Geometry: final body of the model. Coordinates: model frame, mm. A direction names the side the tool comes from. Round coordinates to 2 decimals unless told otherwise and drop trailing zeros. Order: outer loops, then holes, each group sorted by start corner. A loop starts at its lowest first (then second) coordinate and runs counter-clockwise, first axis right, second up. Notation, with made-up numbers: (-27, 54.25) - (22, 54.25) arc R7 cw to (22, 67.25) - close; hole circle Ø10 at (-12, -36). An arc over 180 degrees is marked (long way). Put each result on its own line as item: value. Start each with the question number.
(1) Access query for faces 4 (the face through (208, 44, 6)), 5 (the face through (411.7, 106.6, 3)). Directions: +Z, -Z, +X, -X, +Y, -Y. A direction counts if a zero-diameter tool reaches every point of the face in a straight line with its end or side. Return the directions, or none.
(2) Pull-direction query (X, two-part tool) for faces 1 (the face through (334.87, 80.88, 2.96)), 2 (the face through (443.46, 91.16, 2.96)), 3 (the face through (-72.19, 134.884, 2.958)); classes: released by +X, released by -X, zero draft, split by the parting line, or undercut.
(3) Pin query (flat end, axial travel): P1, Ø1, axis at x = 92, z = 3, coming from the -Y side; P2, Ø2, axis at y = 35, z = 4, coming from the -X side; P3, Ø1.5, axis at x = 399.5, z = 2, coming from the -Y side. Return the tip coordinate at first contact, or that it passes through.
(4) Material intervals for L1, parallel to Y at x = 436.5, z = 2.75; L2, parallel to X at y = 141, z = 2; L3, parallel to X at y = 142, z = 4, sorted ascending. Write a range as [from, to].
(5) Section A-A (x = 363). Output: boundary loops of the cut face in (y, z), and give its area (3 significant figures).
(6) Section B-B (y = 143.5). Output: boundary loops of the cut face in (x, z).
from build123d import *

# Parameters (mm, degrees)
BOSS_EXTRU_3_DEPTH = 6
CONG_1_R           = 60


with BuildPart() as part:
    # Esquisse3 → Boss.-Extru.3 (new body)
    with BuildSketch(Plane(origin=(-3.638307048, 7.762911288, 0), x_dir=(0.984807753012208, -0.1736481776669307, 0), z_dir=(0, 0, 1))):
        with BuildLine():
            Line((-71.559692406, 137.419515489), (-65.127612513, 98.953577983))
            Line((-65.127612513, 98.953577983), (-46.578471081, 103.06810738))
            Line((-46.578471081, 103.06810738), (-41.164616612, 78.661342338))
            Line((-41.164616612, 78.661342338), (-38.235804807, 79.311004874))
            Line((-38.235804807, 79.311004874), (-40.632352311, 90.115131983))
            Line((-40.632352311, 90.115131983), (-35.750999303, 91.197902877))
            Line((-35.750999303, 91.197902877), (-20.829774243, 61.686423244))
            add(Edge.make_bspline(
                [(38.37456384, 38.513359507), (16.587805448, 35.939302498), (-7.762740615, 43.297007319), (-20.829774243, 61.686423244)],
                knots=[0, 0, 0, 0, 1, 1, 1, 1], degree=3))
            Line((38.37456384, 38.513359507), (40.525402219, 28.816939468))
            Line((40.525402219, 28.816939468), (43.463887608, 29.421342988))
            Line((43.463887608, 29.421342988), (41.519581302, 38.186674133))
            Line((41.519581302, 38.186674133), (76.331388066, 41.811327195))
            Line((76.331388066, 41.811327195), (139.998021134, 54.909412313))
            Line((139.998021134, 54.909412313), (141.283555233, 49.113961235))
            Line((141.283555233, 49.113961235), (144.212367038, 49.763623772))
            Line((144.212367038, 49.763623772), (140.328182794, 67.274322069))
            Line((140.328182794, 67.274322069), (194.592792235, 76.238258828))
            Line((194.592792235, 76.238258828), (196.409589011, 65.389330334))
            Line((196.409589011, 65.389330334), (199.368387691, 65.884820364))
            Line((199.368387691, 65.884820364), (197.394020749, 77.674672735))
            Line((197.394020749, 77.674672735), (220.126485179, 80.877779775))
            Line((220.126485179, 80.877779775), (259.319797933, 92.644471957))
            Line((259.319797933, 92.644471957), (256.937701966, 103.383448575))
            Line((256.937701966, 103.383448575), (289.522543291, 108.601505288))
            Line((289.522543291, 108.601505288), (289.047470566, 113.57888471))
            Line((289.047470566, 113.57888471), (353.181348825, 148.485449649))
            Line((353.181348825, 148.485449649), (354.726860043, 141.517968462))
            Line((354.726860043, 141.517968462), (357.655671848, 142.167630999))
            Line((357.655671848, 142.167630999), (355.923238418, 149.977795812))
            Line((355.923238418, 149.977795812), (428.895770917, 189.525355795))
            Line((428.895770917, 189.525355795), (430.844758526, 180.73892038))
            Line((430.844758526, 180.73892038), (433.739949932, 181.524965365))
            Line((433.739949932, 181.524965365), (436.014097486, 166.698359115))
            Line((436.014097486, 166.698359115), (415.342101107, 152.638893772))
            add(Edge.make_bspline(
                [(415.342101107, 152.638893772), (407.545289081, 148.009298465), (406.957115975, 140.201368924)],
                knots=[0, 0, 0, 1, 1, 1], degree=2))
            Line((406.957115975, 140.201368924), (413.667773401, 110.961548868))
            add(Edge.make_bspline(
                [(413.667773401, 110.961548868), (414.76605418, 103.736931255), (421.786696865, 105.123477115)],
                knots=[0, 0, 0, 1, 1, 1], degree=2))
            Line((421.786696865, 105.123477115), (455.956167923, 112.702873372))
            Line((455.956167923, 112.702873372), (457.472047174, 105.86897916))
            Line((457.472047174, 105.86897916), (159.709513668, 39.819954639))
            Line((159.709513668, 39.819954639), (-11.137841622, 1.922973356))
            Line((-11.137841622, 1.922973356), (-96.082570909, 93.62571577))
            Line((-96.082570909, 93.62571577), (-82.90301036, 133.504271207))
            Line((-82.90301036, 133.504271207), (-71.559692406, 137.419515489))
        make_face()
    extrude(amount=BOSS_EXTRU_3_DEPTH)

    # Congé1
    cong_1_edges = [part.edges().sort_by_distance(p)[0] for p in [
        (-14.27301901, 11.590736258, 3),
    ]]
    fillet(cong_1_edges, radius=CONG_1_R)


solid = part.part
Checks:
1. face 4: +Z, +X, -X, +Y, -Y
1. face 5: +Z, -Z, +Y
2. face 1: undercut
2. face 2: released by +X
2. face 3: released by -X
3. P1: stops at y = 16.22
3. P2: stops at x = -29.7
3. P3: stops at y = 29.67
4. L1: y = [31.32, 38.33], [88.03, 114.88]
4. L2: x = [-68.9, -50.38]
4. L3: x = [-68.36, -50.37]
5. outline: (28.11, 0) - (90.33, 0) - (90.33, 6) - (28.11, 6) - close
5. area: 373 mm²
6. outline: (-67.55, 0) - (-50.35, 0) - (-50.35, 6) - (-67.55, 6) - close
